from build123d import *

# Parameters (mm, degrees)
F0_R     = 2
F1_DEPTH = 3


with BuildPart() as f1:
    # F0 (on Top) → F1 (new body)
    with BuildSketch(Plane.XY):
        with BuildLine():
            Line((-37.5, -5), (37.5, -5))
            Line((37.5, -5), (37.5, -2.131387))
            Line((37.5, -2.131387), (32.50913, -1.9993))
            ThreePointArc((32.50913, -1.9993), (30.562048, -0.004567), (32.5, 1.999037))
            ThreePointArc((32.5, 1.999037), (32.562172, 2), (32.624343, 1.999029))
            Line((32.624343, 1.999029), (37.5, 1.998715))
            Line((37.5, 1.998715), (37.5, 5))
            Line((37.5, 5), (-37.5, 5))
            Line((-37.5, 5), (-37.5, 1.939646))
            Line((-37.5, 1.939646), (-32.523661, 1.992048))
            ThreePointArc((-32.523661, 1.992048), (-30.346636, 0.067762), (-32.388344, -1.999541))
            Line((-32.388344, -1.999541), (-37.5, -1.999541))
            Line((-37.5, -1.999541), (-37.5, -5))
        make_face()
        with Locations((-27.437957, 0)):
            Circle(F0_R, mode=Mode.SUBTRACT)
        with Locations((-22.437957, 0)):
            Circle(F0_R, mode=Mode.SUBTRACT)
        with Locations((-17.437957, 0)):
            Circle(F0_R, mode=Mode.SUBTRACT)
        with Locations((-12.437957, 0)):
            Circle(F0_R, mode=Mode.SUBTRACT)
        with Locations((-7.437957, 0)):
            Circle(F0_R, mode=Mode.SUBTRACT)
        with BuildLine():
            ThreePointArc((-0.437957, 0), (-2.437957, -2), (-4.437957, 0))
            ThreePointArc((-4.437957, 0), (-2.437957, 2), (-0.437957, 0))
        make_face(mode=Mode.SUBTRACT)
        with Locations((2.562043, 0)):
            Circle(F0_R, mode=Mode.SUBTRACT)
        with Locations((7.562043, 0)):
            Circle(F0_R, mode=Mode.SUBTRACT)
        with Locations((12.562043, 0)):
            Circle(F0_R, mode=Mode.SUBTRACT)
        with Locations((17.562043, 0)):
            Circle(F0_R, mode=Mode.SUBTRACT)
        with Locations((22.562043, 0)):
            Circle(F0_R, mode=Mode.SUBTRACT)
        with Locations((27.562043, 0)):
            Circle(F0_R, mode=Mode.SUBTRACT)
        with BuildLine():
            ThreePointArc((32.624343, 1.999029), (32.562172, 2), (32.5, 1.999037))
            Line((32.5, 1.999037), (32.624343, 1.999029))
        make_face()
    extrude(amount=F1_DEPTH)


solid = f1.part
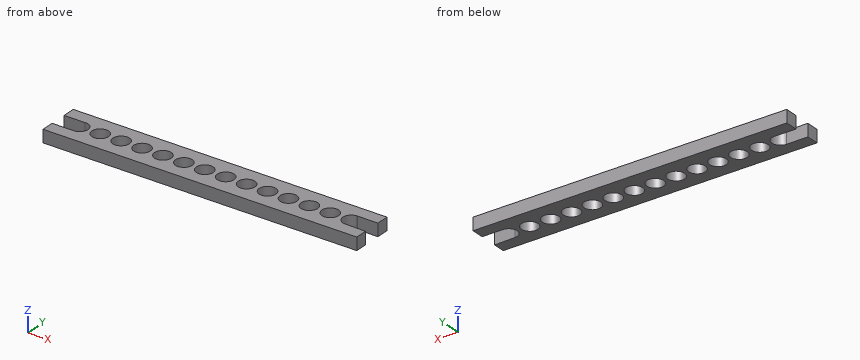
Verification items for the finished model (mm, model axes). Give positions to 0.01 mm unless a question says otherwise; leave off trailing zeros. Loops run counter-clockwise (first coordinate to the right, second up) from the corner with the lowest first, then second, coordinate; pieces in that order, holes last.
1) Sectioned sample at D-D, the plane x = 23. Enter the section's corners in (y, z), then the cut area to 3 significant figures.
2) Sectioned sample at A-A, the plane z = 0.7. Count the separate pieces of the cut face and the enclosed holes in it, then the cut area to 3 significant figures.
3) Sectioned sample at B-B, the plane x = -2.5. Enter the section's corners in (y, z), then the cut area to 3 significant figures.
4) Thickness scan on line 1 along Y through (x, z) = (-34, 0.25); line 2 along Y through (x, z) = (-6, 1.5). Record the ranges inside material, lowest first.
Answers:
1. outline: (-5, 0) - (-1.95, 0) - (-1.95, 3) - (-5, 3) - close; (1.95, 0) - (5, 0) - (5, 3) - (1.95, 3) - close
1. area: 18.3 mm2
2. separate pieces: 1
2. enclosed holes: 12
2. area: 546 mm2
3. outline: (-5, 0) - (-2, 0) - (-2, 3) - (-5, 3) - close; (2, 0) - (5, 0) - (5, 3) - (2, 3) - close
3. area: 18.0 mm2
4. line 1: y = -5 to -2, 1.98 to 5
4. line 2: y = -5 to -1.39, 1.39 to 5
